Autodesk Inventor part; units mm, degrees
ref_plane "YZ Plane" through (0, 0, 0) normal (1, 0, 0) x (0, 1, 0)
ref_plane "XZ Plane" through (0, 0, 0) normal (0, 1, 0) x (-1, 0, 0)
ref_plane "XY Plane" through (0, 0, 0) normal (0, 0, 1) x (1, 0, 0)
sketch "Sketch1" plane through (0, 0, 0) normal (0, 1, 0) x (-1, 0, 0)
  line L0 (0, 0) -> (-80, 0)
  line L1 (-80, 0) -> (-80, -50)
  line L2 (-80, -50) -> (0, -50)
  line L3 (0, -50) -> (0, 0)
  dimension "d0" = 80
  dimension "d1" = 50
extrude "Extrusion1" add sketch "Sketch1" along normal blind 2.5
sketch "Sketch2" plane through (0, 2.5, 0) normal (0, 1, 0) x (1, 0, 0)
  circle A0 centre (12.5, 7.5) radius 2
  circle A1 centre (67.5, 7.5) radius 2
  circle A2 centre (12.5, 42.5) radius 2
  circle A3 centre (67.5, 42.5) radius 2
  line L0 (0, 0) -> (80, 0)
  line L1 (0, 50) -> (0, 0)
  dimension "d4" = 4
  dimension "d5" = 4
  dimension "d6" = 4
  dimension "d7" = 4
  dimension "d8" = 55
  dimension "d9" = 35
  dimension "d10" = 7.5
  dimension "d11" = 12.5
sketch "Sketch3" plane through (80, 0, 0) normal (1, 0, 0) x (0, 0, -1)
  line L0 (35, 10) -> (15, 10)
  line L1 (35, 10) -> (35, 2.5)
  line L2 (15, 10) -> (15, 2.5)
  line L3 (0, 2.5) -> (50, 2.5)
  line L4 (16.5, 8.5) -> (33.5, 8.5)
  line L5 (33.5, 8.5) -> (33.5, 2.5)
  line L6 (16.5, 8.5) -> (16.5, 2.5)
  point P0 (0, 0)
  point P1 (25, 10)
  point P2 (25, 2.5)
  point P3 (25, 8.5)
  dimension "d14" = 20
  dimension "d15" = 7.5
  dimension "d16" = 7.5
  dimension "d17" = 17
  dimension "d18" = 1.5
extrude "Extrusion3" add sketch "Sketch3" against normal blind 77.5 contours L1 L3 L5 L4 L6 L2 L0
sketch "Sketch4" plane through (80, 10, -15) normal (0, 1, 0) x (1, 0, 0)
  line L0 (-57.5, 15) -> (-22.5, 15)
  line L1 (-22.5, 15) -> (-22.5, 5)
  line L2 (-22.5, 5) -> (-57.5, 5)
  line L3 (-57.5, 5) -> (-57.5, 15)
  line L4 (-77.5, 0) -> (-77.5, 20)
  point P0 (-80, -15)
  point P1 (-57.5, 10)
  point P2 (-77.5, 10)
  dimension "d21" = 35
  dimension "d22" = 10
  dimension "d23" = 20
extrude "Extrusion4" cut sketch "Sketch4" against normal blind 1.5
fillet "Fillet2" radius 1 6 edges at (41.25, 10, -15) (41.25, 10, -35) (22.5, 9.25, -30) (57.5, 9.25, -30) (57.5, 9.25, -20) (22.5, 9.25, -20)
fillet "Fillet3" radius 2 4 edges at (80, 1.25, 0) (80, 1.25, -50) (0, 1.25, 0) (0, 1.25, -50)
hole "Hole1" at (67.5, 2.5, -42.5) at (67.5, 2.5, -7.5) at (12.5, 2.5, -7.5) at (12.5, 2.5, -42.5) direction (0, -1, 0) diameter 4 end through all countersink diameter 8 countersink angle 90
fillet "Fillet4" radius 1 4 edges at (67.5, 2.5, -46.5) (12.5, 2.5, -46.5) (67.5, 2.5, -11.5) (12.5, 2.5, -11.5)
fillet "Fillet5" radius 1.5 9 edges at (79.4142, 2.5, -0.5858) (80, 2.5, -8.5) (0.5858, 2.5, -0.5858) (0, 2.5, -25) (0.5858, 2.5, -49.4142) (40, 2.5, -50) (79.4142, 2.5, -49.4142) (80, 2.5, -41.5) (40, 2.5, 0)
fillet "Fillet6" radius 0.5 10 edges at (2.5, 9.7071, -34.7071) (2.5, 5.75, -35) (2.5, 9.7071, -15.2929) (2.5, 5.75, -15) (2.5, 10, -25) (80, 9.7071, -15.2929) (80, 5.75, -15) (80, 9.7071, -34.7071) (80, 5.75, -35) (80, 10, -25)
properties part number "Latch Base" material "Steel"
Design review of the part built by this model. Coordinates are the model's own, in mm. A direction names the side the tool comes from. Round coordinates to 2 decimals unless told otherwise and drop trailing zeros. Write each loop counter-clockwise with the first axis right and the second up, starting at its lowest first coordinate (ties: lowest second). Pieces come first, ordered by that corner, then holes.
Item 1: For faces 1 (the cylindrical face through (79.57, 2.05, -8.66)), 2 (the flat face through (42, 6, -35)), 3 (the flat face through (42, 6, -16.5)), list the 3-axis set-ups (+Z, -Z, +X, -X, +Y, -Y) from which the entire face can be reached by the end or side of a thin tool; tool diameter is ignored.
Item 2: We need section D-D on x = 42.5. Write out the cut boundary in (y, z).
Item 3: We need section C-C on z = -28. Write out the cut boundary in (x, y), and give its area (3 significant figures).
Item 4: The part is to be moulded in two halves that separate along Y. For faces 4 (the cylindrical face through (39.47, 2.05, -0.43)), 5 (the cylindrical face through (0.57, 0.51, -0.6)), 6 (the flat face through (42, 6, -33.5)), say which applies: +Y half, -Y half, draft (parallel to the pull), parting line (faces both ways), or undercut.
Item 5: We need section A-A on x = 67.5. State how many separate pieces and enclosed holes the cut face has, and give its area (3 significant figures).
Item 6: For probe 1 along X at (y, z) = (0.25, -42.5); probe 2 along Z at (x, y) = (67.5, 0.25); probe 3 along Z at (x, y) = (23.5, 7), list the stretches that pass through material, from the lowest coordinate up.
Item 7: We need section B-B on y = 3.5. Write out the cut boundary in (x, z).
Item 8: Clearance check with flat-ended pins moving along their axes: pin 1 Ø3 at (x, y) = (57, 6.5) entering from -Z; pin 2 Ø1.2 at (x, y) = (44, 9) entering from +Z; pin 3 Ø5 at (x, z) = (12.5, -7.5) entering from +Y; pin 4 Ø2.5 at (x, z) = (12.5, -42.5) entering from +Y. State where each tip first meets the part, or that it passes through.
Returned:
1. face 1: +Z, +X, +Y
1. face 2: -Z, +X, -X, +Y
1. face 3: +X, -X
2. outline: (0, -50) - (1, -50) arc R1.5 ccw to (2.5, -48.5) - (2.5, -35) - (9, -35) arc R1 ccw to (10, -34) - (10, -30) - (8.5, -30) - (8.5, -33.5) - (2.5, -33.5) - (2.5, -16.5) - (8.5, -16.5) - (8.5, -20) - (10, -20) - (10, -16) arc R1 ccw to (9, -15) - (2.5, -15) - (2.5, -1.5) arc R1.5 ccw to (1, 0) - (0, 0) - close
3. outline: (0, 0) - (80, 0) - (80, 2.5) - (1.5, 2.5) arc R1.5 ccw to (0, 1) - close; (2.5, 8.5) - (22.5, 8.5) - (22.5, 10) - (3, 10) arc R0.5 ccw to (2.5, 9.5) - close; (57.5, 8.5) - (80, 8.5) - (80, 9.5) arc R0.5 ccw to (79.5, 10) - (57.5, 10) - close
3. area: 263 mm2
4. face 4: +Y half
4. face 5: draft
4. face 6: undercut
5. separate pieces: 3
5. enclosed holes: 1
5. area: 144 mm2
6. probe 1: x = 0 to 10.5, 14.5 to 65.5, 69.5 to 80
6. probe 2: z = -50 to -44.5, -40.5 to -9.5, -5.5 to 0
6. probe 3: z = -35 to -33.5, -16.5 to -15
7. outline: (2.5, -34.5) arc R0.5 ccw to (3, -35) - (79.5, -35) arc R0.5 ccw to (80, -34.5) - (80, -33.5) - (2.5, -33.5) - close; (2.5, -16.5) - (80, -16.5) - (80, -15.5) arc R0.5 ccw to (79.5, -15) - (3, -15) arc R0.5 ccw to (2.5, -15.5) - close
8. pin 1: stops at z = -35
8. pin 2: stops at z = -15
8. pin 3: stops at y = 1
8. pin 4: passes through
